```python
from build123d import *

# Parameters (mm, degrees)
ESQUISSE1_R                  = 10
ESQUISSE1_R_2                = 5
BOSS_EXTRU_1_DEPTH           = 20
BOSS_EXTRU_2_START           = -10
ESQUISSE2_R                  = 5
BOSS_EXTRU_2_DEPTH           = 10
ENL_V_MAT_EXTRU_1_DEPTH      = 33.050741021
ENL_V_MAT_EXTRU_1_DEPTH_BACK = 33.050741021
ESQUISSE3_R                  = 3.25
CONG_1_R                     = 5


with BuildPart() as part:
    # Esquisse1 → Boss.-Extru.1 (new body)
    with BuildSketch(Plane.XY):
        Circle(ESQUISSE1_R)
        Circle(ESQUISSE1_R_2, mode=Mode.SUBTRACT)
    extrude(amount=BOSS_EXTRU_1_DEPTH)

    # Esquisse2 → Boss.-Extru.2 (add)
    with BuildSketch(Plane.XY.offset(20).offset(BOSS_EXTRU_2_START)):
        Polygon((22.5, -5.226497308), (22.5, 5.226497308), (12.5, 11), (-12.5, 11), (-22.5, 5.226497308), (-22.5, -5.226497308), (-12.5, -11), (12.5, -11), align=None)
        Circle(ESQUISSE2_R, mode=Mode.SUBTRACT)
    extrude(amount=BOSS_EXTRU_2_DEPTH)

    # Esquisse3 → Enlèv. mat.-Extru.1 (cut, two sides: drawn at the far end of the back side and taken through both)
    with BuildSketch(Plane.XY.offset(20).offset(-ENL_V_MAT_EXTRU_1_DEPTH_BACK)):
        with Locations((15, 0)):
            Circle(ESQUISSE3_R)
        with Locations((-15, 0)):
            Circle(ESQUISSE3_R)
    extrude(amount=ENL_V_MAT_EXTRU_1_DEPTH + ENL_V_MAT_EXTRU_1_DEPTH_BACK, mode=Mode.SUBTRACT)

    # Congé1
    cong_1_edges = [part.edges().sort_by_distance(p)[0] for p in [
        (22.5, -5.226497308, 15),
        (12.5, -11, 15),
        (-12.5, -11, 15),
        (-22.5, -5.226497308, 15),
        (-22.5, 5.226497308, 15),
        (-12.5, 11, 15),
        (12.5, 11, 15),
        (22.5, 5.226497308, 15),
    ]]
    fillet(cong_1_edges, radius=CONG_1_R)


solid = part.part
```
Work out the finished part from the listing and answer in its coordinate system (mm). A direction names the side the tool comes from. Round coordinates to 2 decimals unless told otherwise and drop trailing zeros. Order: outer loops, then holes, each group sorted by start corner. A loop starts at its lowest first (then second) coordinate and runs counter-clockwise, first axis right, second up.
Q1. Find the intervals of material crossed by line 1 along X through (y, z) = (3.5, 1.5); line 2 along X through (y, z) = (3, 9.5); line 3 along X through (y, z) = (-3, 10.25), in increasing order.
Solution:
line 1: x = -9.37 to -3.57, 3.57 to 9.37
line 2: x = -9.54 to -4, 4 to 9.54
line 3: x = -22.46 to -16.25, -13.75 to -4, 4 to 13.75, 16.25 to 22.46
Q2. A cutting plane is placed at D-D, the plane y = 3.75. Determine the outline of the cut face in (x, z).
Solution:
outline: (-22.3, 10) - (-9.27, 10) - (-9.27, 0) - (-3.31, 0) - (-3.31, 20) - (-22.3, 20) - close; (3.31, 0) - (9.27, 0) - (9.27, 10) - (22.3, 10) - (22.3, 20) - (3.31, 20) - close
Q3. A cutting plane is placed at C-C, the plane z = 12. Determine the outline of the cut face in (x, y).
Solution:
outline: (-22.5, -2.34) arc R5 ccw to (-20, -6.67) - (-13.66, -10.33) arc R5 ccw to (-11.16, -11) - (11.16, -11) arc R5 ccw to (13.66, -10.33) - (20, -6.67) arc R5 ccw to (22.5, -2.34) - (22.5, 2.34) arc R5 ccw to (20, 6.67) - (13.66, 10.33) arc R5 ccw to (11.16, 11) - (-11.16, 11) arc R5 ccw to (-13.66, 10.33) - (-20, 6.67) arc R5 ccw to (-22.5, 2.34) - close; hole circle Ø6.5 at (-15, 0); hole circle Ø10 at (0, 0); hole circle Ø6.5 at (15, 0)
Q4. The mould has two halves that part along X. Classify faces 1 (the cylindrical face through (12.472, 10.825, 15.07)), 2 (the cylindrical face through (-18.247, 0.143, 14.93)), 3 (the flat face through (-16.875, -8.474, 14.93)): pulls with the +X half, pulls with the -X half, needs draft (parallel to the pull), parting line crosses it, or undercut.
Solution:
face 1: pulls with the +X half
face 2: undercut
face 3: pulls with the -X half
Q5. A tool of negligible diameter and unlimited length cuts with its end or side. For faces 4 (the flat face through (0, 11, 15)), 5 (the cylindrical face through (-2.17, -9.76, 4.93)), from which of +Z, -Z, +X, -X, +Y, -Y can it reach the whole face along a straight path? Write none if from no direction.
Solution:
face 4: +Z, -Z, +X, -X, +Y
face 5: -Z
Q6. A cutting plane is placed at A-A, the plane y = 0. Determine the outline of the cut face in (x, z).
Solution:
outline: (-22.5, 10) - (-18.25, 10) - (-18.25, 20) - (-22.5, 20) - close; (-11.75, 10) - (-10, 10) - (-10, 0) - (-5, 0) - (-5, 20) - (-11.75, 20) - close; (5, 0) - (10, 0) - (10, 10) - (11.75, 10) - (11.75, 20) - (5, 20) - close; (18.25, 10) - (22.5, 10) - (22.5, 20) - (18.25, 20) - close
Q7. Given pin 1 Ø6 at (y, z) = (-5, 4.5) entering from +X; pin 2 Ø6 at (x, y) = (0, 0) entering from -Z; pin 3 Ø3 at (y, z) = (2, 5.5) entering from -X; pin 4 Ø5 at (y, z) = (-7, 12.5) entering from -X, each flat-ended and moving along its own axis, determine where each tip first touches the part or whether it passes through.
Solution:
pin 1: stops at x = 9.8
pin 2: passes through
pin 3: stops at x = -9.99
pin 4: stops at x = -22.01
Q8. A cutting plane is placed at B-B, the plane x = 0. Determine the outline of the cut face in (y, z).
Solution:
outline: (-11, 10) - (-10, 10) - (-10, 0) - (-5, 0) - (-5, 20) - (-11, 20) - close; (5, 0) - (10, 0) - (10, 10) - (11, 10) - (11, 20) - (5, 20) - close
